Verification items for the finished model (mm, model axes). A direction names the side the tool comes from. Round coordinates to 2 decimals unless told otherwise and drop trailing zeros. Order: outer loops, then holes, each group sorted by start corner. A loop starts at its lowest first (then second) coordinate and runs counter-clockwise, first axis right, second up. Notation, with made-up numbers: (59, 22.5) -> (104, 22.5) arc R15 ccw to (104, 45.5) -> close; hole circle Ø2 at (2, 70.25). An arc over 180 degrees is marked (long way). Return JSON: item names as keys, results as strings. Group by question number.
Item 1: Depth check by flat-ended pin: pin 1 Ø3 at (y, z) = (16, 44.5) entering from -X; pin 2 Ø16.5 at (x, y) = (-63.5, 10) entering from -Z; pin 3 Ø3 at (x, z) = (9, -3) entering from +Y; pin 4 Ø12 at (x, z) = (0, 0) entering from +Y. Enter the tip coordinate at first touch or a pass-through.
Item 2: Sectioned sample at D-D on z = -3. Record the cut outline in (x, y).
Item 3: Sectioned sample at C-C on x = 0. Record the cut outline in (y, z), plus the area to 3 significant figures.
Item 4: Sectioned sample at A-A on z = 38. Record the cut outline in (x, y), plus the area to 3 significant figures.
Item 5: Draft check along Z on faces 4 (the cylindrical face through (-49.113, 7.395, 17.635)), 5 (the flat face through (-21, 15, 21)), 6 (the cylindrical face through (-9.76, 24.86, -2.17)). Enter one of: pulls with the +Z half, pulls with the -Z half, needs draft (parallel to the pull), parting line crosses it, or undercut.
Item 6: Sectioned sample at B-B on y = 24. Record the cut outline in (x, z), plus the area to 3 significant figures.
Item 7: Scan lines: probe 1 along X at (y, z) = (8, 40); probe 2 along X at (y, z) = (25, 0); probe 3 along Y at (x, z) = (-18, 16.5). Record each from-to range of solid material in increasing order. Write a range as from..to.
Item 8: Access from +Z, -Z, +X, -X, +Y, -Y to the whole of each face (thin tool, end or side, straight path). Record for faces 1 (the flat face through (-21, 0, 21)), 2 (the cylindrical face through (-19.524, 24.86, -4.336)), 3 (the cylindrical face through (-39, 8, 40)).
```python
from build123d import *

# Parameters (mm, degrees)
BOSS_EXTRUDE1_DEPTH = 15
SKETCH2_R           = 20
SKETCH2_R_2         = 10
BOSS_EXTRUDE2_DEPTH = 20
SKETCH5_R           = 7.5
CUT_EXTRUDE1_DEPTH  = 116.866302263
CUT_EXTRUDE2_DEPTH  = 116.866302263


with BuildPart() as part:
    # Sketch1 → Boss-Extrude1 (new body)
    with BuildSketch(Plane(origin=(0, 0, 0), x_dir=(1, 0, 0), z_dir=(0, 1, 0))):
        with BuildLine():
            Line((-85, -55), (5, -55))
            ThreePointArc((5, -55), (14.16042736, -51.877986807), (19.507658043, -43.811542745))
            Line((19.507658043, -43.811542745), (29.015316087, -7.623085489))
            ThreePointArc((29.015316087, -7.623085489), (8.389479092, 28.803066513), (-28.570577696, 9.149977603))
            ThreePointArc((-28.570577696, 9.149977603), (-49.525739839, -17.897965522), (-82.966509351, -25.138475321))
            ThreePointArc((-82.966509351, -25.138475321), (-99.965341128, -38.980899952), (-85, -55))
        make_face()
    extrude(amount=BOSS_EXTRUDE1_DEPTH)

    # Sketch2 → Boss-Extrude2 (add)
    with BuildSketch(Plane(origin=(0, 15, 0), x_dir=(1, 0, 0), z_dir=(0, 1, 0))):
        with Locations(Location((0, 0, 0), (0, 0, 270))):
            Circle(SKETCH2_R)
        with Locations(Location((0, 0, 0), (0, 0, 270))):
            Circle(SKETCH2_R_2, mode=Mode.SUBTRACT)
    extrude(amount=BOSS_EXTRUDE2_DEPTH)

    # Sketch5 → Cut-Extrude1 (cut, through all)
    with BuildSketch(Plane(origin=(0, 15, 0), x_dir=(1, 0, 0), z_dir=(0, 1, 0))):
        with Locations(Location((5, -40, 0), (0, 0, 270))):
            Circle(SKETCH5_R)
    extrude(amount=-CUT_EXTRUDE1_DEPTH, mode=Mode.SUBTRACT)

    # Sketch6 → Cut-Extrude2 (cut, through all)
    with BuildSketch(Plane(origin=(0, 15, 0), x_dir=(1, 0, 0), z_dir=(0, 1, 0))):
        with BuildLine():
            Line((-85, -34), (-45, -34))
            ThreePointArc((-45, -34), (-39, -40), (-45, -46))
            Line((-45, -46), (-85, -46))
            ThreePointArc((-85, -46), (-91, -40), (-85, -34))
        make_face()
    extrude(amount=-CUT_EXTRUDE2_DEPTH, mode=Mode.SUBTRACT)


solid = part.part
```
Recorded:
{
 "1": {"pin 1": "x = -99.61", "pin 2": "z = 21", "pin 3": "y = 35", "pin 4": "y = 15"},
 "2": {"outline": "(-31, 0) -> (29.85, 0) -> (29.85, 15) -> (19.77, 15) -> (19.77, 35) -> (9.54, 35) -> (9.54, 15) -> (-9.54, 15) -> (-9.54, 35) -> (-19.77, 35) -> (-19.77, 15) -> (-31, 15) -> close"},
 "3": {"outline": "(0, -30) -> (15, -30) -> (15, -20) -> (35, -20) -> (35, -10) -> (15, -10) -> (15, 10) -> (35, 10) -> (35, 20) -> (15, 20) -> (15, 34.41) -> (0, 34.41) -> close; (0, 45.59) -> (15, 45.59) -> (15, 55) -> (0, 55) -> close", "area": "1,510 mm²"},
 "4": {"outline": "(-99.87, 0) -> (-90.66, 0) -> (-90.66, 15) -> (-99.87, 15) -> close; (-39.34, 0) -> (-2.23, 0) -> (-2.23, 15) -> (-39.34, 15) -> close; (12.23, 0) -> (21.03, 0) -> (21.03, 15) -> (12.23, 15) -> close", "area": "827 mm²"},
 "5": {"face 4": "pulls with the -Z half", "face 5": "needs draft", "face 6": "undercut"},
 "6": {"outline": "circle Ø40 at (0, 0); hole circle Ø20 at (0, 0)", "area": "942 mm²"},
 "7": {"probe 1": "-100..-91, -39..-2.5, 12.5..20.51", "probe 2": "-20..-10, 10..20", "probe 3": "0..15"},
 "8": {"face 1": "+Z, -Z, +X, -X, -Y", "face 2": "+Y", "face 3": "+Y, -Y"}
}
